from build123d import *

# Parameters (mm, degrees)
F0_R     = 6.35
F1_DEPTH = 11.176
F0_R_2   = 14.2875
F2_DEPTH = 41.148
F3_R     = 3.048


with BuildPart() as f1:
    # F0 (on Top) → F1 (new body)
    with BuildSketch(Plane.XY):
        with BuildLine():
            ThreePointArc((-11.017324, 22.886209), (13.515176, 21.505813), (25.4, 0))
            ThreePointArc((25.4, 0), (13.515176, -21.505813), (-11.017324, -22.886209))
            Line((-11.017324, -22.886209), (40.256642, -47.569279))
            ThreePointArc((40.256642, -47.569279), (56.337591, -49.833259), (68.321377, -38.873725))
            Line((68.321377, -38.873725), (68.321377, 0))
            Line((68.321377, 0), (68.321377, 38.873725))
            ThreePointArc((68.321377, 38.873725), (56.337591, 49.833259), (40.256642, 47.569279))
            Line((40.256642, 47.569279), (-11.017324, 22.886209))
        make_face()
        with Locations((50.8, -28.575)):
            Circle(F0_R, mode=Mode.SUBTRACT)
        with Locations((50.8, 28.575)):
            Circle(F0_R, mode=Mode.SUBTRACT)
    extrude(amount=F1_DEPTH)

    # F0 (on Top) → F2 (join)
    with BuildSketch(Plane.XY):
        with BuildLine():
            ThreePointArc((-11.017324, -22.886209), (13.515176, -21.505813), (25.4, 0))
            ThreePointArc((25.4, 0), (13.515176, 21.505813), (-11.017324, 22.886209))
            ThreePointArc((-11.017324, 22.886209), (-25.4, 0), (-11.017324, -22.886209))
        make_face()
        Circle(F0_R_2, mode=Mode.SUBTRACT)
    extrude(amount=F2_DEPTH)

    # F3
    f3_edges = [f1.edges().sort_by_distance(p)[0] for p in [
        (11.017324, -22.886209, 41.148),
    ]]
    fillet(f3_edges, radius=F3_R)


solid = f1.part
Input: part model. Units: mm. Frame: model coordinates. Give positions to 0.01 mm unless a question says otherwise; leave off trailing zeros. Order: outer loops, then holes, each group sorted by start corner. A loop starts at its lowest first (then second) coordinate and runs counter-clockwise, first axis right, second up.
Q1. Section A-A on x = 50.8. Output: boundary loops of the cut face in (y, z) (3 decimals).
Checked values:
outline: (-50.686, 0) - (-34.925, 0) - (-34.925, 11.176) - (-50.686, 11.176) - close; (-22.225, 0) - (22.225, 0) - (22.225, 11.176) - (-22.225, 11.176) - close; (34.925, 0) - (50.686, 0) - (50.686, 11.176) - (34.925, 11.176) - close
Q2. Contact query for flat-ended pins moving along their axis: pin 1 Ø3 at (y, z) = (20.5, 18) entering from -X; pin 2 Ø5 at (x, z) = (2, 29.5) entering from +Y; pin 3 Ø6 at (y, z) = (-11.5, 33) entering from +X. Output: stop coordinate, or through.
Checked values:
pin 1: stops at x = -16.86
pin 2: stops at y = 25.4
pin 3: stops at x = 23.94
Q3. Draft query along Y for faces 1 (the cylindrical face through (-14.274, 0.628, 20.286)), 2 (the flat face through (68.321, -1, 6)), 3 (the cylindrical face through (56.113, -49.901, 5.51)). Return one class per face: +Y half, -Y half, draft (parallel to the pull), parting line (faces both ways), or undercut.
Checked values:
face 1: undercut
face 2: draft
face 3: -Y half
Q4. Section B-B on z = 21. Output: boundary loops of the cut face in (x, y) (1 decimal).
Checked values:
outline: circle Ø50.8 at (0, 0); hole circle Ø28.6 at (0, 0)
Q5. Section C-C on x = 30.5. Output: boundary loops of the cut face in (y, z), and give its area (3 significant figures).
Checked values:
outline: (-42.87, 0) - (42.87, 0) - (42.87, 11.18) - (-42.87, 11.18) - close
area: 958 mm2
Q6. Ray query, probe 1 along Y at (x, z) = (0, 26); probe 2 along Y at (x, z) = (50, 3); probe 3 along Z at (x, y) = (2.5, 28.5). Return the intervals inside material, ascending.
Checked values:
probe 1: y = -25.4 to -14.29, 14.29 to 25.4
probe 2: y = -50.67 to -34.87, -22.28 to 22.28, 34.87 to 50.67
probe 3: z = 0 to 11.18
Q7. Section D-D on x = 61. Output: boundary loops of the cut face in (y, z), and give its area (3 significant figures).
Checked values:
outline: (-47.66, 0) - (47.66, 0) - (47.66, 11.18) - (-47.66, 11.18) - close
area: 1,070 mm2
